Input: dimensioned drawing with shaded views. Units: mm. Origin: part minimum x, y, z. A direction names the side the tool comes from. Give positions to 0.01 mm unless a question says otherwise; leave off trailing zeros. Write each loop counter-clockwise with the first axis right and the second up, starting at its lowest first coordinate (ties: lowest second). Pieces come first, ordered by that corner, then holes. Notation, with made-up numbers: (25, 68) - (42, 68) arc R28 ccw to (42, 98) - close; hole circle Ø6 at (71, 12). An arc over 180 degrees is marked (long way). Answer as a JSON object with one key per item and string values. Group by question number.
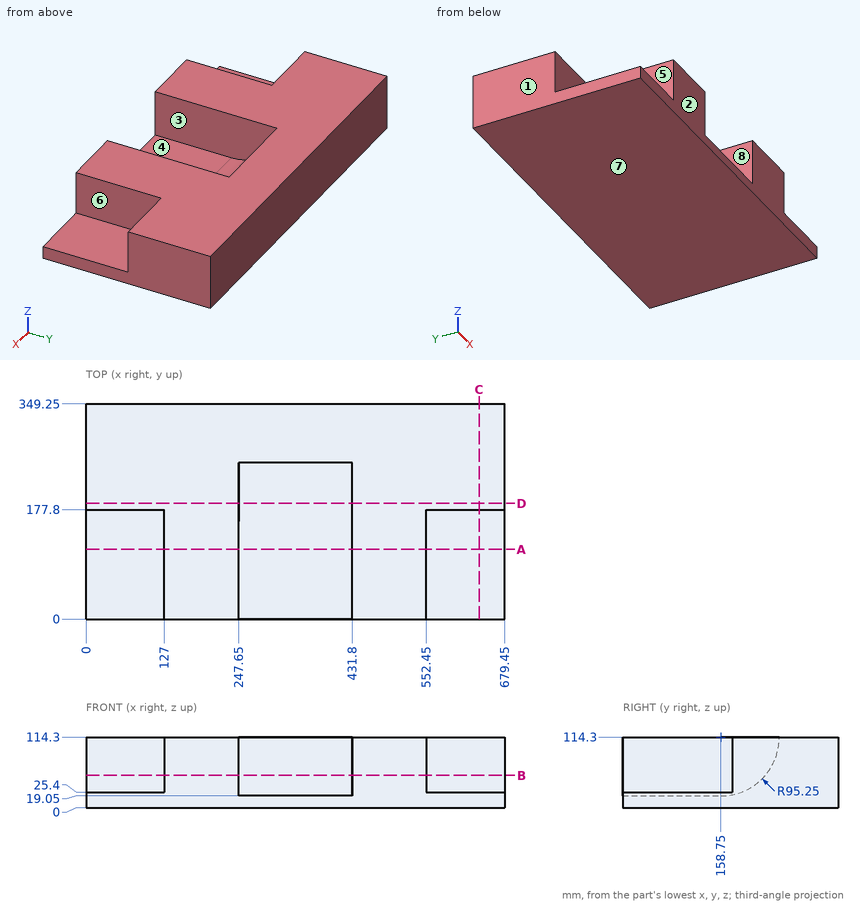
Q1. Section D-D on y = 188. Return the cut outline in (x, z).
Q2. Reachability of the marked faces 5, 6, 7 and 8 from +Z, -Z, +X, -X, +Y, -Y: full face, straight path, thin tool, end or side. Return the list, or none.
Q3. Section A-A on y = 113.5. Return the cut outline in (x, z).
Q4. Ray query, probe 1 along X at (y, z) = (102.5, 59.5); probe 2 along X at (y, z) = (223, 66); probe 3 along Z at (x, y) = (335, 50.5). Return the intervals inside material, ascending. Write a range as [from, to].
Q5. Section C-C on x = 638. Return the cut outline in (y, z), then the cut area to 3 significant figures.
Q6. First-contact query: pin 1 Ø1.5 at (x, y) = (308.5, 80.5) entering from +Z; pin 2 Ø6 at (x, y) = (422.5, 225.5) entering from +Z; pin 3 Ø3 at (x, y) = (269.5, 169) entering from +Z. Flat tips, straight axial feed; report the tip coordinate or a pass-through.
Q7. Section B-B on z = 52.5. Return the cut outline in (x, y), then the cut area to 3 significant figures.
Q8. Draft query along X for the marked faces 1, 2, 3 and 4. Return one class per face: released by +X, released by -X, zero draft, split by the parting line, or undercut.
Taken from the geometry:
{
 "1": {"outline": "(0, 0) - (679.45, 0) - (679.45, 114.3) - (431.8, 114.3) - (431.8, 23.65) - (247.65, 23.65) - (247.65, 114.3) - (0, 114.3) - close"},
 "2": {"face 5": "+Z, -X, -Y", "face 6": "+Z, +X, -Y", "face 7": "-Z, +X, -X, +Y, -Y", "face 8": "+Z, -Y"},
 "3": {"outline": "(0, 0) - (679.45, 0) - (679.45, 25.4) - (552.45, 25.4) - (552.45, 114.3) - (431.8, 114.3) - (431.8, 19.05) - (247.65, 19.05) - (247.65, 114.3) - (127, 114.3) - (127, 25.4) - (0, 25.4) - close"},
 "4": {"probe 1": "x = [127, 247.65], [431.8, 552.45]", "probe 2": "x = [0, 247.65], [431.8, 679.45]", "probe 3": "z = [0, 19.05]"},
 "5": {"outline": "(0, 0) - (349.25, 0) - (349.25, 114.3) - (177.8, 114.3) - (177.8, 25.4) - (0, 25.4) - close", "area": "24,100 mm²"},
 "6": {"pin 1": "stops at z = 19.05", "pin 2": "stops at z = 49.43", "pin 3": "stops at z = 19.78"},
 "7": {"outline": "(0, 177.8) - (127, 177.8) - (127, 0) - (247.65, 0) - (247.65, 231.23) - (431.8, 231.23) - (431.8, 0) - (552.45, 0) - (552.45, 177.8) - (679.45, 177.8) - (679.45, 349.25) - (0, 349.25) - close", "area": "150,000 mm²"},
 "8": {"face 1": "released by -X", "face 2": "zero draft", "face 3": "undercut", "face 4": "undercut"}
}
